```python
from build123d import *

# Parameters (mm, degrees)
SKETCH_R     = 60
SKETCH_R_2   = 6
PAD_DEPTH    = 5
PAD001_DEPTH = 5


with BuildPart() as part:
    # Sketch → Pad (new body)
    with BuildSketch(Plane.XZ):
        Circle(SKETCH_R)
        Circle(SKETCH_R_2, mode=Mode.SUBTRACT)
    extrude(amount=PAD_DEPTH)

    # Sketch001 → Pad001 (new body)
    with BuildSketch(Plane.XZ):
        with BuildLine():
            ThreePointArc((10.908712, -59), (0, 60), (-10.908712, -59))
            Line((-10.908712, -19.994713), (-10.908712, -59))
            Line((-16.031858, -19.994713), (-10.908712, -19.994713))
            ThreePointArc((-20, -16.079947), (-18.790704, -18.822669), (-16.031858, -19.994713))
            Line((-20, -16.079947), (-20, 20.005287))
            Line((-20, 20.005287), (20, 20.005287))
            Line((20, 20.005287), (20, -19.994713))
            Line((20, -19.994713), (10.908712, -19.994713))
            Line((10.908712, -19.994713), (10.908712, -59))
        make_face()
    extrude(amount=-PAD001_DEPTH)


solid = part.part
```
Verification items for the finished model (mm, model axes). A direction names the side the tool comes from. Give positions to 0.01 mm unless a question says otherwise; leave off trailing zeros. Loops run counter-clockwise (first coordinate to the right, second up) from the corner with the lowest first, then second, coordinate; pieces in that order, holes last. Notation, with made-up numbers: M 44,27.25 L 74,27.25 A37 ccw 74,63.25 Z; hole C -15.75,-29 d1. An arc over 180 degrees is marked long. Return JSON: item names as keys, results as strings.
1) Mould release check, pull along X, two halves, no side actions. Record for faces 1 (the flat face through (12, -5, 1)), 2 (the flat face through (20, 2, 0)): released by +X, released by -X, zero draft, split by the parting line, or undercut.
Findings:
{"face 1": "zero draft", "face 2": "undercut"}
2) Section check A-A, the plane z = 0. Enter the section's corners in (x, y).
Findings:
{"outline": "M -60,-5 L -6,-5 L -6,0 L -20,0 L -20,5 L -60,5 Z; M 6,-5 L 60,-5 L 60,5 L 20,5 L 20,0 L 6,0 Z"}
3) Section check B-B, the plane x = 0. Enter the section's corners in (y, z), and give its area (3 significant figures).
Findings:
{"outline": "M -5,-60 L 0,-60 L 0,-6 L -5,-6 Z; M -5,6 L 0,6 L 0,20.01 L 5,20.01 L 5,60 L -5,60 Z", "area": "740 mm2"}
4) Material ranges on L1, parallel to Z at x = 0, y = -2.25; L2, parallel to X at y = 1.75, z = -45.5; L3, parallel to X at y = 2.5, z = -37.5, recorded low to high. Write a range as [from, to].
Findings:
{"L1": "z = [-60, -6], [6, 60]", "L2": "x = [-39.11, -10.91], [10.91, 39.11]", "L3": "x = [-46.84, -10.91], [10.91, 46.84]"}
5) Gauge pin test, flat ends, axial feed: P1, Ø1.5, axis at y = 3.5, z = -4.5, coming from the +X side; P2, Ø1.5, axis at x = -14, y = 2, coming from the +Z side; P3, Ø12, axis at x = 2, z = -29, coming from the +Y side; P4, Ø7, axis at x = 0, z = 0, coming from the +Y side. Record the tip position at first contact, or that the pin passes through.
Findings:
{"P1": "stops at x = 59.88", "P2": "stops at z = 58.52", "P3": "stops at y = 0", "P4": "passes through"}
6) Tool access check on faces 3 (the flat face through (-10.909, 2, -39)), 4 (the flat face through (-20, 2, 2)), 5 (the cylindrical face through (-6, -2, 0)). Record the directions out of +Z, -Z, +X, -X, +Y, -Y that give a thin tool (end or side, any length) a straight path to the whole face; none if there is none.
Findings:
{"face 3": "-Z, +Y", "face 4": "+Y", "face 5": "+Y, -Y"}
7) Section check D-D, the plane x = 13. Enter the section's corners in (y, z), and give its area (3 significant figures).
Findings:
{"outline": "M -5,-58.57 L 5,-58.57 L 5,-19.99 L 0,-19.99 L 0,20.01 L 5,20.01 L 5,58.57 L -5,58.57 Z", "area": "971 mm2"}
8) Section check C-C, the plane y = 2.75. Enter the section's corners in (x, z), and give its area (3 significant figures).
Findings:
{"outline": "M -20,-16.08 L -20,20.01 L 20,20.01 L 20,-19.99 L 10.91,-19.99 L 10.91,-59 A60 ccw long -10.91,-59 L -10.91,-19.99 L -16.03,-19.99 A4.07 cw Z", "area": "8,850 mm2"}
